CAD build for the part. Positions are in the model's coordinates, mm. Face numbers are marked on the shaded views. A direction names the side the tool comes from. Round coordinates to 2 decimals unless told otherwise and drop trailing zeros. Order: outer loops, then holes, each group sorted by start corner. A loop starts at its lowest first (then second) coordinate and runs counter-clockwise, first axis right, second up. Notation, with made-up numbers: M -32.5,9 L 5.5,9 A19 ccw 5.5,27 Z; hole C 61.5,72.25 d3. An arc over 180 degrees is marked long. Put each result on its own line as item: value.
```python
from build123d import *

# Parameters (mm, degrees)
SKETCH_W     = 37.973
SKETCH_H     = 2.286
PAD_DEPTH    = 2.54
PAD001_DEPTH = 1.7
SKETCH002_R  = 1.778
POCKET_DEPTH = 5
SKETCH003_W  = 16
SKETCH003_H  = 20.5
PAD002_DEPTH = 19
SKETCH007_W  = 9.8
SKETCH007_H  = 7.7
PAD004_DEPTH = 10


with BuildPart() as part:
    # Sketch (on Face2 of Binder001) → Pad (new body)
    with BuildSketch(Plane.XY.offset(10.414)):
        with Locations((-20.1295, 2.413)):
            Rectangle(SKETCH_W, SKETCH_H)
    extrude(amount=PAD_DEPTH)

    # Sketch001 (on Face6 of Pad) → Pad001 (join)
    with BuildSketch(Plane.XY.offset(12.954)):
        Polygon((-66.04, 53.34), (-1.27, 53.34), (0, 52.07), (0, 40.903026), (2.54, 37.836974), (2.54, 5.343026), (0, 2.276974), (0, 0.635), (-0.635, 0), (-66.04, 0), align=None)
    extrude(amount=PAD001_DEPTH)

    # Sketch002 (on Face5 of Pad001) → Pocket (cut)
    with BuildSketch(Plane.XY.offset(14.654)):
        with Locations((-52.07, 2.54)):
            Circle(SKETCH002_R)
        with Locations((-50.8, 50.8)):
            Circle(SKETCH002_R)
    extrude(amount=-POCKET_DEPTH, mode=Mode.SUBTRACT)

    # Sketch003 (on Face5 of Pocket) → Pad002 (join)
    with BuildSketch(Plane.XY.offset(14.654)):
        with Locations((-43.7, 38.53)):
            Rectangle(SKETCH003_W, SKETCH003_H)
        with Locations((-22, 38.53)):
            Rectangle(SKETCH003_W, SKETCH003_H)
        with Locations((-43.7, 14.81)):
            Rectangle(SKETCH003_W, SKETCH003_H)
        with Locations((-22, 14.81)):
            Rectangle(SKETCH003_W, SKETCH003_H)
    extrude(amount=PAD002_DEPTH)

    # Sketch007 (on Face5 of Pad002) → Pad004 (join)
    with BuildSketch(Plane.XY.offset(14.654)):
        with Locations((-61.14, 13.55)):
            Rectangle(SKETCH007_W, SKETCH007_H)
    extrude(amount=PAD004_DEPTH)


solid = part.part
```
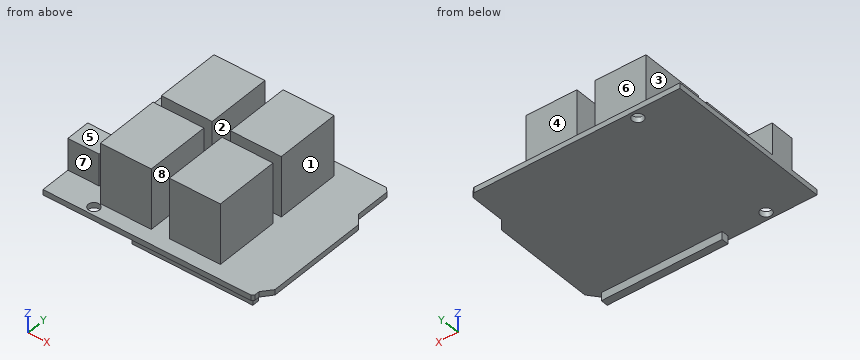
Item 1: Band-saw the part on A-A on z = 29. Give the cut face in (x, y), and give its area (3 significant figures).
Answers below:
outline: M -51.7,4.56 L -35.7,4.56 L -35.7,25.06 L -51.7,25.06 Z; M -51.7,28.28 L -35.7,28.28 L -35.7,48.78 L -51.7,48.78 Z; M -30,4.56 L -14,4.56 L -14,25.06 L -30,25.06 Z; M -30,28.28 L -14,28.28 L -14,48.78 L -30,48.78 Z
area: 1,310 mm²
Item 2: Pin check, flat tips, straight feed: P1, Ø5, axis at x = -60.5, z = 17.5, coming from the -Y side; P2, Ø5, axis at x = -23.5, z = 24, coming from the -Y side; P3, Ø1.4, axis at y = 48.5, z = 14, coming from the +X side; P4, Ø2, axis at x = -52.07, y = 2.54, coming from the -Z side. Stop position of each tip, or through.
Answers below:
P1: y = 9.7
P2: y = 4.56
P3: x = 0
P4: through
Item 3: Band-saw the part on C-C on x = -29. Give the cut face in (y, z).
Answers below:
outline: M 0,12.95 L 1.27,12.95 L 1.27,10.41 L 3.56,10.41 L 3.56,12.95 L 53.34,12.95 L 53.34,14.65 L 48.78,14.65 L 48.78,33.65 L 28.28,33.65 L 28.28,14.65 L 25.06,14.65 L 25.06,33.65 L 4.56,33.65 L 4.56,14.65 L 0,14.65 Z
Item 4: Mould opens along X. For the marked faces 1, 2, 3 and 4 say: pulls with the +X half, pulls with the -X half, needs draft (parallel to the pull), parting line crosses it, or undercut.
Answers below:
face 1: pulls with the +X half
face 2: undercut
face 3: pulls with the -X half
face 4: needs draft
Item 5: Band-saw the part on B-B on z = 15.75. Give the cut face in (x, y).
Answers below:
outline: M -66.04,9.7 L -56.24,9.7 L -56.24,17.4 L -66.04,17.4 Z; M -51.7,4.56 L -35.7,4.56 L -35.7,25.06 L -51.7,25.06 Z; M -51.7,28.28 L -35.7,28.28 L -35.7,48.78 L -51.7,48.78 Z; M -30,4.56 L -14,4.56 L -14,25.06 L -30,25.06 Z; M -30,28.28 L -14,28.28 L -14,48.78 L -30,48.78 Z
Item 6: Tool access for the marked faces 5, 6, 7 and 8: list every direction of +Z, -Z, +X, -X, +Y, -Y with a clear straight run to the whole face (end or side of a thin tool).
Answers below:
face 5: +Z, -X, +Y, -Y
face 6: +Z, +X, -X, +Y
face 7: +Z, -X, -Y
face 8: +Z, +Y, -Y
Item 7: Band-saw the part on D-D on y = 50.8. Give the cut face in (x, z), and give its area (3 significant figures).
Answers below:
outline: M -66.04,12.95 L -52.58,12.95 L -52.58,14.65 L -66.04,14.65 Z; M -49.02,12.95 L 0,12.95 L 0,14.65 L -49.02,14.65 Z
area: 106 mm²
Item 8: Probe line 1 along X through (y, z) = (23.5, 21.25); line 2 along Y through (x, z) = (-38, 21.75); line 3 along Y through (x, z) = (-52.07, 14.15). List the from-to ranges inside material, lowest first. Write a range as [from, to].
Answers below:
line 1: [-51.7, -35.7], [-30, -14]
line 2: [4.56, 25.06], [28.28, 48.78]
line 3: [0, 0.76], [4.32, 49.56], [52.04, 53.34]
